Design review of the part shown in the three views and the two pictorial views. Dimensions are in mm from the part's minimum x, y and z. Round coordinates to 2 decimals unless told otherwise and drop trailing zeros. Loops run counter-clockwise (first coordinate to the right, second up) from the corner with the lowest first, then second, coordinate; pieces in that order, holes last. Notation, with made-up numbers: (-23.5, 87) -> (19.5, 87) arc R25 cw to (19.5, 102) -> close; hole circle Ø3 at (10.25, 14.5). An arc over 180 degrees is marked (long way). Return JSON: item names as keys, results as strings. Group by question number.
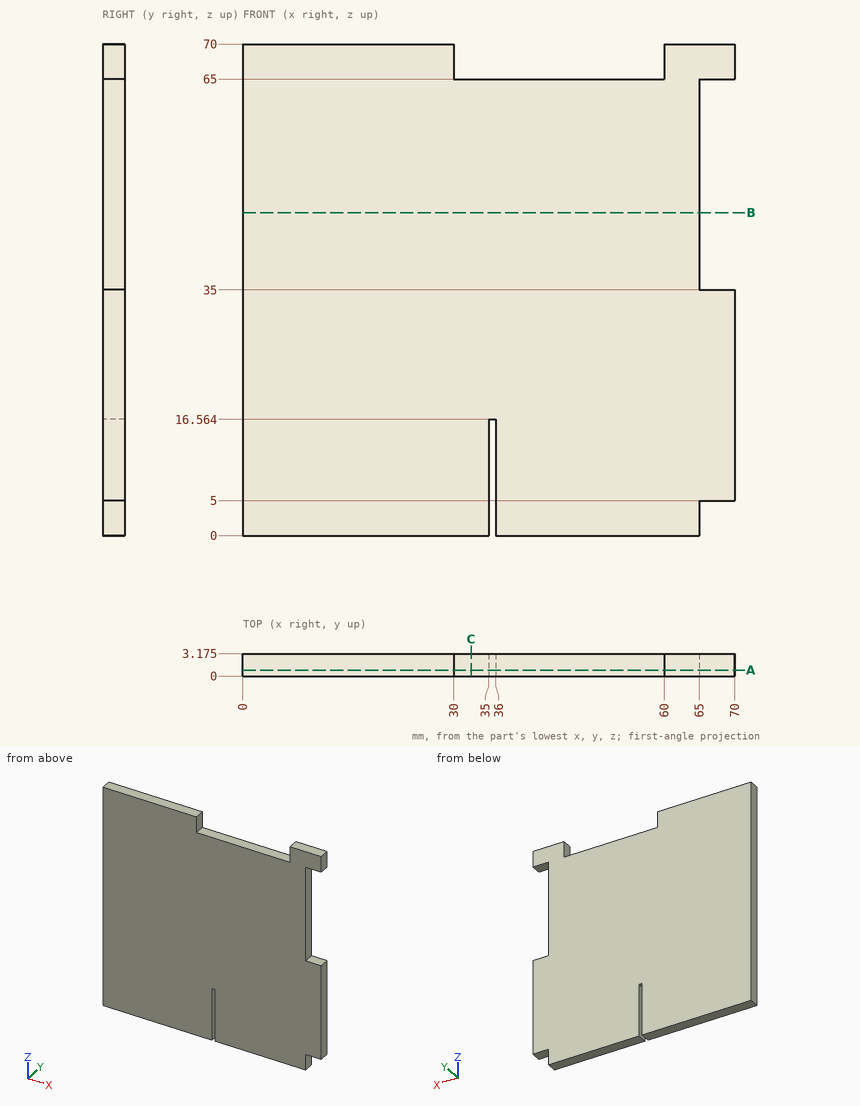
1. We need section B-B, the plane z = 46. Write out the cut boundary in (x, y) (1 decimal), then the cut area to 3 significant figures.
2. We need section C-C, the plane x = 32.5. Write out the cut boundary in (y, z) (1 decimal), then the cut area to 3 significant figures.
3. Wall thickness on line 1 (X direction, y = 1, z = 8); line 2 (X direction, y = 2, z = 4); line 3 (X direction, y = 0.2, z = 38.5): over which ranges is each line inside the solid? List them lowest first.
4. We need section A-A, the plane y = 0.85. Write out the cut boundary in (x, z), then the cut area to 3 significant figures.
5. For P1, Ø1.6, axis at x = 68.5, y = 2.5, coming from the -Z side; P2, Ø1.6, axis at y = 1.5, z = 49, coming from the +X side; P3, Ø1, axis at x = 49.5, y = 1, coming from the +Z side, all flat-tipped, find the tip position at first contact; note any pin that passes through.
Check sheet entries:
{
 "1": {"outline": "(0, 0) -> (65, 0) -> (65, 3.2) -> (0, 3.2) -> close", "area": "206 mm²"},
 "2": {"outline": "(0, 0) -> (3.2, 0) -> (3.2, 65) -> (0, 65) -> close", "area": "206 mm²"},
 "3": {"line 1": "x = 0 to 35, 36 to 70", "line 2": "x = 0 to 35, 36 to 65", "line 3": "x = 0 to 65"},
 "4": {"outline": "(0, 0) -> (35, 0) -> (35, 16.56) -> (36, 16.56) -> (36, 0) -> (65, 0) -> (65, 5) -> (70, 5) -> (70, 35) -> (65, 35) -> (65, 65) -> (70, 65) -> (70, 70) -> (60, 70) -> (60, 65) -> (30, 65) -> (30, 70) -> (0, 70) -> close", "area": "4,560 mm²"},
 "5": {"P1": "stops at z = 5", "P2": "stops at x = 65", "P3": "stops at z = 65"}
}
